from build123d import *

# Parameters (mm, degrees)
SALIENTE_EXTRUIR1_DEPTH = 3
CROQUIS2_R              = 8.5
CORTAR_EXTRUIR1_DEPTH   = 81.972978651
CROQUIS3_RX             = 9.378712311
CROQUIS3_RY             = 8.5
CORTAR_EXTRUIR2_DEPTH   = 3
CROQUIS4_W              = 43
CROQUIS4_H              = 16.468521704
CORTAR_EXTRUIR3_DEPTH   = 80.113842029
REDONDEO1_R             = 3
CROQUIS5_W              = 150
CROQUIS5_H              = 1
CORTAR_EXTRUIR4_DEPTH   = 80.113842155


with BuildPart() as part:
    # Croquis1 → Saliente-Extruir1 (new body)
    with BuildSketch(Plane.XY):
        Polygon((-75, -19), (-75, -25), (75, -25), (75, -19), (72, -19), (72, -4), (75, -4), (75, 10), (72, 10), (72, 25), (-72, 25), (-72, 10), (-75, 10), (-75, -4), (-72, -4), (-72, -19), align=None)
    extrude(amount=SALIENTE_EXTRUIR1_DEPTH)

    # Croquis2 → Cortar-Extruir1 (cut, through all)
    with BuildSketch(Plane(origin=(0, 2.342305324, -10.565456544), x_dir=(1, 0, 0), z_dir=(0, -0.4226182617407, 0.9063077870366497))):
        with Locations(Location((-13, 11.342305324, 0), (0, 0, 90))):
            Circle(CROQUIS2_R)
        with Locations(Location((13, 11.342305324, 0), (0, 0, 90))):
            Circle(CROQUIS2_R)
    extrude(amount=CORTAR_EXTRUIR1_DEPTH, mode=Mode.SUBTRACT)

    # Croquis3 → Cortar-Extruir2 (cut)
    with BuildSketch(Plane.XY):
        with Locations(Location((-13, 8.531478296), (0, 0, 90))):
            Ellipse(CROQUIS3_RX, CROQUIS3_RY)
        with Locations(Location((-13, 9.930401271), (0, 0, 90))):
            Ellipse(CROQUIS3_RX, CROQUIS3_RY)
        with Locations(Location((-13, 9.930401271), (0, 0, 90))):
            Ellipse(CROQUIS3_RX, CROQUIS3_RY)
        with Locations(Location((-13, 8.531478296), (0, 0, 90))):
            Ellipse(CROQUIS3_RX, CROQUIS3_RY)
        with Locations(Location((13, 9.930401271), (0, 0, 90))):
            Ellipse(CROQUIS3_RX, CROQUIS3_RY)
        with Locations(Location((13, 8.531478296), (0, 0, 90))):
            Ellipse(CROQUIS3_RX, CROQUIS3_RY)
        with Locations(Location((13, 8.531478296), (0, 0, 90))):
            Ellipse(CROQUIS3_RX, CROQUIS3_RY)
        with Locations(Location((13, 9.930401271), (0, 0, 90))):
            Ellipse(CROQUIS3_RX, CROQUIS3_RY)
        with Locations(Location((13, 8.531478296), (0, 0, 90))):
            Ellipse(CROQUIS3_RX, CROQUIS3_RY)
        with Locations(Location((13, 9.930401271), (0, 0, 90))):
            Ellipse(CROQUIS3_RX, CROQUIS3_RY)
        with Locations(Location((-13, 8.531478296), (0, 0, 90))):
            Ellipse(CROQUIS3_RX, CROQUIS3_RY)
        with Locations(Location((-13, 9.930401271), (0, 0, 90))):
            Ellipse(CROQUIS3_RX, CROQUIS3_RY)
    extrude(amount=CORTAR_EXTRUIR2_DEPTH, mode=Mode.SUBTRACT)

    # Croquis4 → Cortar-Extruir3 (cut, through all)
    with BuildSketch(Plane.XY):
        with Locations((0, 16.765739148)):
            Rectangle(CROQUIS4_W, CROQUIS4_H)
    extrude(amount=CORTAR_EXTRUIR3_DEPTH, mode=Mode.SUBTRACT)

    # Redondeo1
    redondeo1_edges = [part.edges().sort_by_distance(p)[0] for p in [
        (4.5, 8.531478296, 1.5000003),
        (-4.5, 8.531478296, 1.5000003),
        (21.5, 25, 1.5),
        (-21.5, 25, 1.5),
    ]]
    fillet(redondeo1_edges, radius=REDONDEO1_R)

    # Croquis5 → Cortar-Extruir4 (cut, through all)
    with BuildSketch(Plane.XY):
        with Locations((0, -24.5)):
            Rectangle(CROQUIS5_W, CROQUIS5_H)
    extrude(amount=CORTAR_EXTRUIR4_DEPTH, mode=Mode.SUBTRACT)


solid = part.part
Check sheet for the modelled part. Datum: model origin and axes. Units: mm. A direction names the side the tool comes from. Round coordinates to 2 decimals unless told otherwise and drop trailing zeros. Loops run counter-clockwise (first coordinate to the right, second up) from the corner with the lowest first, then second, coordinate; pieces in that order, holes last. Notation, with made-up numbers: (-11, 24.25) - (46, 24.25) arc R32 ccw to (46, 57.25) - close; hole circle Ø7 at (17, 40). An arc over 180 degrees is marked (long way). Answer as CSV lines item,"result". Start each with the question number.
Item 1: Section check A-A (y = 15). Record the boundary of the cut face in (x, z).
Item 2: Scan lines: line 1 (X direction, y = 16.5, z = 2.2); line 2 (X direction, y = 0.5, z = 1); line 3 (X direction, y = 0, z = 2.4). Record each from-to range of solid material in increasing order. Write a range as [from, to].
Item 3: Set-up check for faces 1 (the flat face through (-72, 18, 1)), 2 (the flat face through (0, 8.531, 1)), 3 (the flat face through (74, -19, 1)), 4 (the flat face through (-73, -19, 1)), 5 (the flat face through (72, 17, 1)): record each of +Z, -Z, +X, -X, +Y, -Y from which the full face is reachable in a straight line by a thin tool's end or side.
Item 4: Depth check by flat-ended pin: P1, Ø1.5, axis at y = 15, z = 1.5, coming from the -X side; P2, Ø0.9, axis at x = -73.5, z = 2, coming from the +Y side; P3, Ø0.9, axis at y = 15, z = 1.5, coming from the +X side. Enter the tip coordinate at first touch or a pass-through.
Item 5: Release check for a two-part mould opening along X. For faces 6 (the flat face through (73, -4, 1)), 7 (the flat face through (21.5, 15, 1)), 8 (the flat face through (-75, -21, 1)) record: +X half, -X half, draft (parallel to the pull), parting line (faces both ways), or undercut.
Item 6: Section check C-C (y = 4.5). Count the separate pieces of the cut face and the enclosed holes in it, and give its area (3 significant figures).
Item 7: Section check B-B (y = -10). Record the boundary of the cut face in (x, z).
Report:
1,outline,"(-72, 0) - (-21.5, 0) - (-21.5, 3) - (-72, 3) - close; (21.5, 0) - (72, 0) - (72, 3) - (21.5, 3) - close"
2,line 1,"x = [-72, -21.5], [21.5, 72]"
2,line 2,"x = [-75, -17.39], [-8.61, 8.61], [17.39, 75]"
2,line 3,"x = [-75, -16.53], [-9.47, 9.47], [16.53, 75]"
3,face 1,"+Z, -Z, -X, +Y"
3,face 2,"+Z, -Z, +Y"
3,face 3,"+Z, -Z, +X"
3,face 4,"+Z, -Z, -X"
3,face 5,"+Z, -Z, +X, +Y"
4,P1,"stops at x = -72"
4,P2,"stops at y = 10"
4,P3,"stops at x = 72"
5,face 6,"draft"
5,face 7,"undercut"
5,face 8,"-X half"
6,separate pieces,"3"
6,enclosed holes,"0"
6,area,"358 mm2"
7,outline,"(-72, 0) - (72, 0) - (72, 3) - (-72, 3) - close"
